```python
from build123d import *

# Parameters (mm, degrees)
BOSS_EXTRUDE1_DEPTH = 20
SKETCH3_W           = 10
SKETCH3_H           = 20
BOSS_EXTRUDE2_DEPTH = 20
SKETCH4_R           = 2.5
CUT_EXTRUDE1_DEPTH  = 30


with BuildPart() as part:
    # Sketch2 → Boss-Extrude1 (new body)
    with BuildSketch(Plane(origin=(0, 0, 0), x_dir=(1, 0, 0), z_dir=(0, 1, 0))):
        Polygon((-283.5, 163.678801315), (283.5, 163.678801315), (0, -327.357602631), align=None)
    extrude(amount=BOSS_EXTRUDE1_DEPTH)

    # Sketch3 → Boss-Extrude2 (add)
    with BuildSketch(Plane(origin=(141.75, 0, 81.839400658), x_dir=(0.5, 0, -0.866025404), z_dir=(0.866025404, 0, 0.5))):
        with Locations((-10, 10)):
            Rectangle(SKETCH3_W, SKETCH3_H)
        with Locations((10, 10)):
            Rectangle(SKETCH3_W, SKETCH3_H)
    boss_extrude2 = extrude(amount=BOSS_EXTRUDE2_DEPTH)

    # Sketch4 → Cut-Extrude1 (cut)
    with BuildSketch(Plane(origin=(-7.5, 0, 12.990381057), x_dir=(0.866025404, 0, 0.5), z_dir=(-0.5, 0, 0.866025404))):
        with Locations((173.678801315, 10)):
            Circle(SKETCH4_R)
    cut_extrude1 = extrude(amount=-CUT_EXTRUDE1_DEPTH, mode=Mode.SUBTRACT)

    # Mirror1: Boss-Extrude2, Cut-Extrude1 across plane
    add(boss_extrude2.mirror(Plane(origin=(0, 0, 0), x_dir=(-0.866025404, 0, 0.5), z_dir=(0.5, 0, 0.866025404))))
    add(cut_extrude1.mirror(Plane(origin=(0, 0, 0), x_dir=(-0.866025404, 0, 0.5), z_dir=(0.5, 0, 0.866025404))), mode=Mode.SUBTRACT)

    # Mirror1 at the second plane: Boss-Extrude2, Cut-Extrude1 across plane
    add(boss_extrude2.mirror(Plane(origin=(0, 0, 0), x_dir=(0, 0, 1), z_dir=(1, 0, 0))))
    add(cut_extrude1.mirror(Plane(origin=(0, 0, 0), x_dir=(0, 0, 1), z_dir=(1, 0, 0))), mode=Mode.SUBTRACT)


solid = part.part
```
Here's how the part is built. I have some questions about the finished solid (model axes, mm). A direction names the side the tool comes from. Coordinates: 2 decimals unless noted, no trailing zeros. Order: outer loops, then holes, each group sorted by start corner. A loop starts at its lowest first (then second) coordinate and runs counter-clockwise, first axis right, second up.
1) Will these pins go through, and if not, where does the flat tip stop? pin 1 (10 mm diameter, centred on y = 11, z = -177, fed in from +X); pin 2 (2 mm diameter, centred on x = 146, y = 7.5, fed in from +Z); pin 3 (3 mm diameter, centred on y = 10, z = -173.68, fed in from +X); pin 4 (2 mm diameter, centred on x = 98.5, y = 6.5, fed in from -Z).
2) Imagine slicing it at B-B on x = -181. List the corners of the cut face in (y, z) for me.
3) We'd pull the mould along X, two halves only. Please class faces 1 (the face through (5, 12, -176)), 2 (the face through (4, 0, 11)), 3 (the face through (-15, 12, -171)): +X half, -X half, draft (parallel to the pull), parting line (faces both ways), or undercut.
4) Imagine slicing it at A-A on z = -86. List the corners of the cut face in (x, y) for me.
5) I need wall thicknesses on line 1 (Z direction, x = -155.5, y = 10.5); line 2 (Z direction, x = -12.5, y = 10); line 3 (Z direction, x = -8, y = 10). Which ranges of each line are inside material? Lowest first, please.
6) Which directions (+Z, -Z, +X, -X, +Y, -Y) give clear straight access to the entire face, cutting with the end or side of a thin tool? Please do faces 4 (the face through (-154.71, 12.08, 83.55)), 5 (the face through (-155.865, 12.082, 72.668)), 6 (the face through (147, 10, -163.679)), 7 (the face through (-140.865, 12.082, 98.649)), 8 (the face through (159.71, 12.08, 74.89)).
Response values:
1. pin 1: stops at x = 15
1. pin 2: stops at z = 102.19
1. pin 3: passes through
1. pin 4: stops at z = -163.68
2. outline: (0, -163.68) - (20, -163.68) - (20, 13.86) - (0, 13.86) - close
3. face 1: undercut
3. face 2: draft
3. face 3: -X half
4. outline: (-238.65, 0) - (238.65, 0) - (238.65, 20) - (-238.65, 20) - close
5. line 1: z = -163.68 to 58.02, 72.46 to 73.12, 82.92 to 84, 95.55 to 98.02
5. line 2: z = -183.68 to -176.18, -171.18 to 305.71
5. line 3: z = -183.68 to -176.18, -171.18 to 313.5
6. face 4: +Y, -Y
6. face 5: -X, +Y, -Y
6. face 6: -Z, +X, +Y, -Y
6. face 7: +Z, +Y, -Y
6. face 8: +X, +Y, -Y
